```python
from build123d import *
from build123d.topology import SkipClean

# Parameters (mm, degrees)
SKETCH1_R           = 2.85
BOSS_EXTRUDE1_DEPTH = 1
SKETCH2_R           = 10
BOSS_EXTRUDE2_DEPTH = 2
BOSS_EXTRUDE3_START = 1
BOSS_EXTRUDE3_DEPTH = 1
CUT_EXTRUDE1_DEPTH  = 1
BOSS_EXTRUDE4_START = 5
BOSS_EXTRUDE4_DEPTH = 5
BOSS_EXTRUDE5_START = 10
BOSS_EXTRUDE5_DEPTH = 10


with BuildPart() as part:
    # Sketch1 → Boss-Extrude1 (new body)
    with BuildSketch(Plane.XY):
        Circle(SKETCH1_R)
    extrude(amount=BOSS_EXTRUDE1_DEPTH)

    # Sketch2 → Boss-Extrude2 (add)
    with BuildSketch(Plane.XY.offset(1)):
        Circle(SKETCH2_R)
    extrude(amount=BOSS_EXTRUDE2_DEPTH)

    # Sketch3 → Boss-Extrude3 (add)
    with BuildSketch(Plane(origin=(0, 0, 1), x_dir=(-1, 0, 0), z_dir=(0, 0, -1)).offset(BOSS_EXTRUDE3_START)):
        with BuildLine():
            Line((-9.986209241, 0.525), (9.986209241, 0.525))
            ThreePointArc((9.986209241, 0.525), (10, 0), (9.986209241, -0.525))
            Line((9.986209241, -0.525), (-9.986209241, -0.525))
            ThreePointArc((-9.986209241, -0.525), (-10, 0), (-9.986209241, 0.525))
        make_face()
    extrude(amount=-BOSS_EXTRUDE3_DEPTH)

    # Sketch4 → Cut-Extrude1 (cut)
    with BuildSketch(Plane(origin=(0, 0, 0), x_dir=(-1, 0, 0), z_dir=(0, 0, -1))):
        with BuildLine():
            ThreePointArc((0.5, 2.805797569), (0, 2.85), (-0.5, 2.805797569))
            Line((-0.5, 2.805797569), (0, 1.939772166))
            Line((0, 1.939772166), (0.5, 2.805797569))
        make_face()
    extrude(amount=-CUT_EXTRUDE1_DEPTH, mode=Mode.SUBTRACT)

    # Sketch5 → Boss-Extrude4 (add)
    with SkipClean():  # the faces are left unmerged after this step: merging them gives an invalid solid
        with BuildSketch(Plane(origin=(0, 0, 0), x_dir=(-1, 0, 0), z_dir=(0, 0, -1)).offset(BOSS_EXTRUDE4_START)):
            with BuildLine():
                ThreePointArc((2.80122741, 0.525), (2.006248985, 2.024219605), (0.5, 2.805797569))
                Line((0.5, 2.805797569), (0, 1.939772166))
                Line((0, 1.939772166), (-0.5, 2.805797569))
                ThreePointArc((-0.5, 2.805797569), (-2.006248985, 2.024219605), (-2.80122741, 0.525))
                ThreePointArc((-2.80122741, 0.525), (-2.85, 0), (-2.80122741, -0.525))
                ThreePointArc((-2.80122741, -0.525), (0, -2.85), (2.80122741, -0.525))
                ThreePointArc((2.80122741, -0.525), (2.85, 0), (2.80122741, 0.525))
            make_face()
        extrude(amount=-BOSS_EXTRUDE4_DEPTH)

    # Sketch6 → Boss-Extrude5 (add)
    with SkipClean():  # the faces are left unmerged after this step: merging them gives an invalid solid
        with BuildSketch(Plane(origin=(0, 0, 0), x_dir=(-1, 0, 0), z_dir=(0, 0, -1)).offset(BOSS_EXTRUDE5_START)):
            with BuildLine():
                ThreePointArc((-4.469270075, -0.525), (-4.5, 0), (-4.469270075, 0.525))
                Line((-4.469270075, 0.525), (-9.986209241, 0.525))
                ThreePointArc((-9.986209241, 0.525), (-10, 0), (-9.986209241, -0.525))
                Line((-9.986209241, -0.525), (-4.469270075, -0.525))
            make_face()
            with BuildLine():
                ThreePointArc((4.469270075, 0.525), (4.5, 0), (4.469270075, -0.525))
                Line((4.469270075, -0.525), (9.986209241, -0.525))
                ThreePointArc((9.986209241, -0.525), (10, 0), (9.986209241, 0.525))
                Line((9.986209241, 0.525), (4.469270075, 0.525))
            make_face()
        extrude(amount=-BOSS_EXTRUDE5_DEPTH)


solid = part.part
```
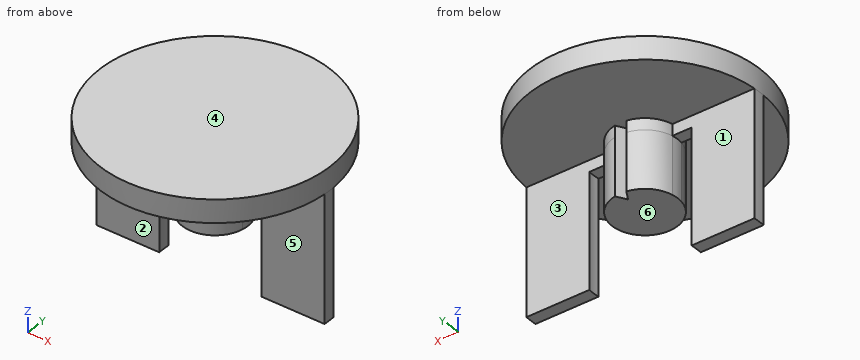
For this review, take the finished solid that the model builds, in its own axes (mm). Face numbers are marked on the shaded views. A direction names the side the tool comes from. Coordinates: 2 decimals unless noted, no trailing zeros. Loops run counter-clockwise (first coordinate to the right, second up) from the corner with the lowest first, then second, coordinate; pieces in that order, holes last.
1. Add section A-A, the plane z = -4.5. Give the boundary of the cut face in (x, y) (3 decimals), then the cut area to 3 significant figures.
2. Insertion check: P1, Ø4, axis at x = -6.5, z = -3.5, coming from the +Y side (3 decimals); P2, Ø10.5, axis at x = -5, y = -7.5, coming from the -Z side; P3, Ø1, axis at x = -5, z = -5.5, coming from the -Y side (3 decimals); P4, Ø1.2, axis at x = -4, y = 0, coming from the -Z side. Each pin has a flat end and moves straight along its axis. Give the tip position at first contact, or say it passes through.
3. Add section C-C, the plane y = 0. Give the boundary of the cut face in (x, z), then the cut area to 4 significant figures.
4. For the marked faces 1, 2, 3 and 4, list the 3-axis set-ups (+Z, -Z, +X, -X, +Y, -Y) from which the entire face can be reached by the end or side of a thin tool; tool diameter is ignored.
5. Add section D-D, the plane x = 8.5. Give the boundary of the cut face in (y, z) (3 decimals).
6. Add section B-B, the plane z = -8.5. Give the boundary of the cut face in (x, y) (3 decimals).
7. Mouldability with a two-part tool opening along X and no side actions: class the marked faces 5 and 6 as +X half, -X half, draft (parallel to the pull), parting line (faces both ways), or undercut.
8. For line 1 (Y direction, x = 5.5, z = -5.5) (3 decimals); line 2 (Z direction, x = -5.5, y = 4.25); line 3 (X direction, y = 6, z = 1.5), list the stretches that pass through material, from the lowest coordinate up.
Result:
1. outline: (-9.986, -0.525) - (-4.469, -0.525) arc R4.5 cw to (-4.469, 0.525) - (-9.986, 0.525) arc R10 ccw to start; (-0.5, 2.806) arc R2.85 ccw (long way) to (0.5, 2.806) - (0, 1.94) - close; (4.469, -0.525) - (9.986, -0.525) arc R10 ccw to (9.986, 0.525) - (4.469, 0.525) arc R4.5 cw to start
1. area: 36.6 mm2
2. P1: stops at y = 0.525
2. P2: stops at z = 1
2. P3: stops at y = -0.525
2. P4: stops at z = -10
3. outline: (-10, -10) - (-4.5, -10) - (-4.5, 0) - (-2.85, 0) - (-2.85, -5) - (2.85, -5) - (2.85, 0) - (4.5, 0) - (4.5, -10) - (10, -10) - (10, 3) - (-10, 3) - close
3. area: 198.5 mm2
4. face 1: -Z, -X, +Y
4. face 2: -Z, -X, -Y
4. face 3: -Z, +X, +Y
4. face 4: +Z, +X, -X, +Y, -Y
5. outline: (-5.268, 1) - (-0.525, 1) - (-0.525, -10) - (0.525, -10) - (0.525, 1) - (5.268, 1) - (5.268, 3) - (-5.268, 3) - close
6. outline: (-9.986, -0.525) - (-4.469, -0.525) arc R4.5 cw to (-4.469, 0.525) - (-9.986, 0.525) arc R10 ccw to start; (4.469, -0.525) - (9.986, -0.525) arc R10 ccw to (9.986, 0.525) - (4.469, 0.525) arc R4.5 cw to start
7. face 5: draft
7. face 6: undercut
8. line 1: y = -0.525 to 0.525
8. line 2: z = 1 to 3
8. line 3: x = -8 to 8
